Here's the drawing with two shaded views (mm, measured from the low corner). I have some questions. A direction names the side the tool comes from. Round coordinates to 2 decimals unless told otherwise and drop trailing zeros. Loops run counter-clockwise (first coordinate to the right, second up) from the corner with the lowest first, then second, coordinate; pieces in that order, holes last. Notation, with made-up numbers: (40.5, -2.75) -> (77.5, -2.75) arc R21 cw to (77.5, 34.25) -> close; hole circle Ø5 at (-4, 69.25). An arc over 180 degrees is marked (long way). Write item = value, one per line.
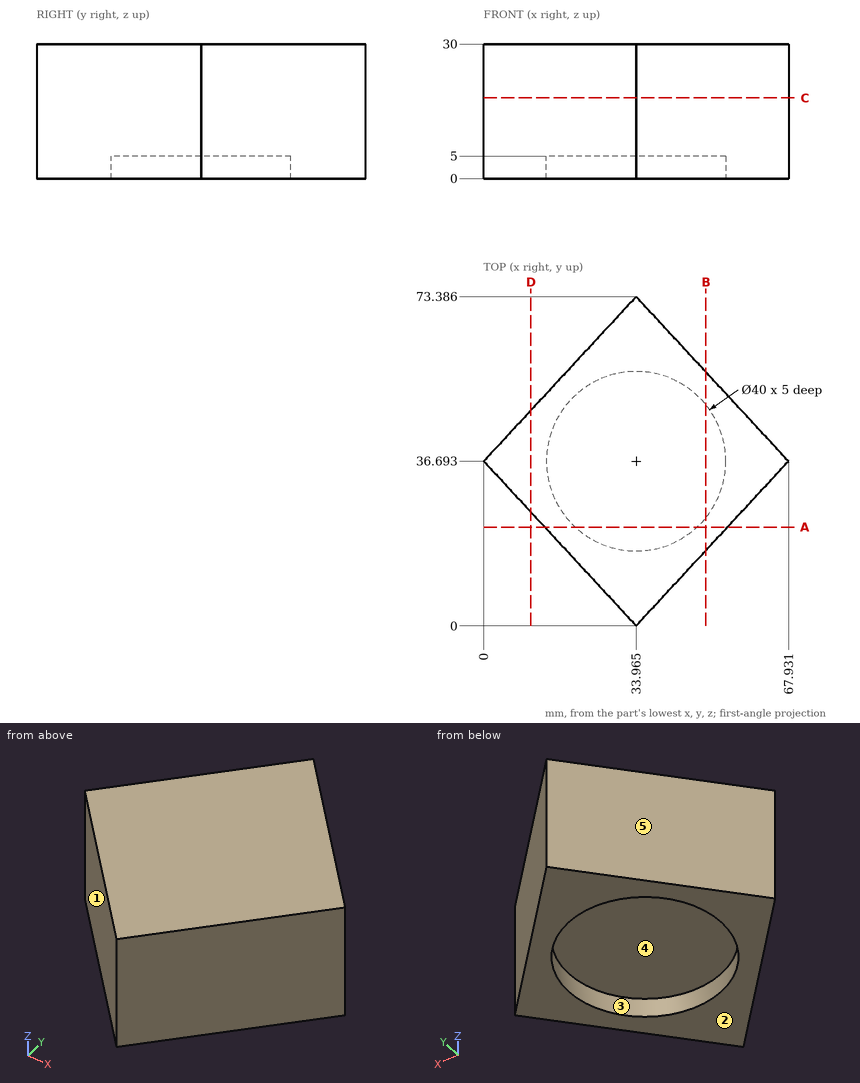
1. We'd pull the mould along Y, two halves only. Please class the marked faces 1, 2 and 3: released by +Y, released by -Y, zero draft, split by the parting line, or undercut.
Entries:
face_1 = released by -Y
face_2 = zero draft
face_3 = undercut
2. I need wall thicknesses on line 1 (X direction, y = 53.5, z = 3.5) (1 decimal); line 2 (X direction, y = 49, z = 4.25); line 3 (Z direction, x = 50, y = 33.5). Which ranges of each line are inside material? Lowest first, please. Write a range as [from, to].
Entries:
line_1 = [15.6, 23.1], [44.8, 52.4]
line_2 = [11.39, 18.2], [49.73, 56.54]
line_3 = [5, 30]
3. Suppose I cut it at D-D, the plane x = 10.5. List the corners of the cut face in (y, z) for me.
Entries:
outline = (25.35, 0) -> (48.04, 0) -> (48.04, 30) -> (25.35, 30) -> close
4. For the marked faces 4 and 5, which set-ups out of +Z, -Z, +X, -X, +Y, -Y let a thin tool reach every point of the face, with its end or its side?
Entries:
face_4 = -Z
face_5 = +Z, -Z, -X, +Y
5. I'm going to push flat-ended pins straight in: pin 1 (1.5 mm diameter, centred on y = 50, z = 17, fed in from +X); pin 2 (6 mm diameter, centred on y = 9, z = 20.5, fed in from -X); pin 3 (20 mm diameter, centred on x = 42, y = 27.5, fed in from -Z); pin 4 (1.5 mm diameter, centred on x = 29.5, z = 11.5, fed in from +Y). Where does each tip first touch, or does it pass through?
Entries:
pin_1 = 56.31
pin_2 = 22.86
pin_3 = 0
pin_4 = 69.37
6. Suppose I cut it at B-B, the plane x = 49.5. List the corners of the cut face in (y, z) for me, and give its area (3 significant figures).
Entries:
outline = (16.78, 0) -> (24.1, 0) -> (24.1, 5) -> (49.29, 5) -> (49.29, 0) -> (56.6, 0) -> (56.6, 30) -> (16.78, 30) -> close
area = 1,070 mm²
7. Suppose I cut it at C-C, the plane z = 18. List the corners of the cut face in (x, y) for me (1 decimal), and give its area (3 significant figures).
Entries:
outline = (0, 36.7) -> (34, 0) -> (67.9, 36.7) -> (34, 73.4) -> close
area = 2,490 mm²
8. Suppose I cut it at A-A, the plane y = 22. List the corners of the cut face in (x, z) for me (1 decimal).
Entries:
outline = (13.6, 0) -> (20.4, 0) -> (20.4, 5) -> (47.5, 5) -> (47.5, 0) -> (54.3, 0) -> (54.3, 30) -> (13.6, 30) -> close
